from build123d import *

# Parameters (mm, degrees)
F0_W     = 180
F0_H     = 110
F1_DEPTH = 35
F0_W_2   = 200
F0_H_2   = 130
F2_DEPTH = 45
F3_R     = 4.99999


# Not quite as in the source:
# - a fillet or chamfer is up to 0.001 mm smaller than in the source, because OpenCascade refuses the exact size


with BuildPart() as f1:
    # F0 (on Front) → F1 (new body)
    with BuildSketch(Plane.XZ):
        Rectangle(F0_W, F0_H)
    extrude(amount=F1_DEPTH)

    # F0 (on Front) → F2 (join)
    with BuildSketch(Plane.XZ):
        Rectangle(F0_W_2, F0_H_2)
        Rectangle(F0_W, F0_H, mode=Mode.SUBTRACT)
    extrude(amount=F2_DEPTH)

    # F3 (radius 5 in the source; OpenCascade refuses exactly that, so slightly less here)
    f3_edges = [f1.edges().sort_by_distance(p)[0] for p in [
        (0, -45, -65),
        (100, -45, 0),
        (0, -45, 65),
        (-100, -45, 0),
        (0, -45, 55),
        (90, -45, 0),
        (0, -45, -55),
        (-90, -45, 0),
        (-100, -22.5, -65),
        (100, -22.5, -65),
        (0, 0, -65),
        (-100, -22.5, 65),
        (-100, 0, 0),
        (100, -22.5, 65),
        (100, 0, 0),
        (0, 0, 65),
    ]]
    fillet(f3_edges, radius=F3_R)


solid = f1.part
For this review, take the finished solid that the model builds, in its own axes (mm). A direction names the side the tool comes from. Round coordinates to 2 decimals unless told otherwise and drop trailing zeros. Put each result on its own line as item: value. Start each with the question number.
1. For faces 1 (the flat face through (90, -37, -1)), 2 (the cylindrical face through (-99, -43, 1)), list the 3-axis set-ups (+Z, -Z, +X, -X, +Y, -Y) from which the entire face can be reached by the end or side of a thin tool; tool diameter is ignored.
2. Insertion check: P1, Ø12, axis at x = -17.5, z = -34.5, coming from the -Y side; P2, Ø4, axis at x = 47, z = -24, coming from the +Y side. Each pin has a flat end and moves straight along its axis. Give the tip position at first contact, or say it passes through.
3. For probe 1 along X at (y, z) = (-40, 2); probe 2 along Z at (x, y) = (53, -36.5); probe 3 along Y at (x, z) = (-59, -12.5), list the stretches that pass through material, from the lowest coordinate up. Write a range as [from, to].
4. Mouldability with a two-part tool opening along X and no side actions: class faces 3 (the flat face through (-100, -22, -1)), 4 (the flat face through (-1, -35, 1)), 5 (the flat face through (100, -22, -1)) as +X half, -X half, draft (parallel to the pull), parting line (faces both ways), or undercut.
Result sheet:
1. face 1: -Y
1. face 2: +Z, -Z, -X, -Y
2. P1: y = -35
2. P2: y = 0
3. probe 1: [-100, -90], [90, 100]
3. probe 2: [-65, -55], [55, 65]
3. probe 3: [-35, 0]
4. face 3: -X half
4. face 4: undercut
4. face 5: +X half
